from build123d import *

# Parameters (mm, degrees)
SKETCH_594_R           = 7.65
CUT_EXTRUDE_2199_DEPTH = 10
CHAMFER_START          = -4.9
CHAMFER_1_2_DEPTH      = 3.6500001
CHAMFER_START_2        = 1.2499999
CHAMFER_1_3_DEPTH      = 3.6500001
CHAMFER_START_3        = -5.4
CHAMFER_1_4_DEPTH      = 3
CHAMFER_START_4        = 2.4
CHAMFER_1_5_DEPTH      = 3
CHAMFER_START_5        = -2.4
CHAMFER_1_6_DEPTH      = 4.8


with BuildPart() as part:
    # Sketch 286 → Revolve 549 (revolve)
    with BuildSketch(Plane.XY, mode=Mode.PRIVATE) as revolve_549_sk:
        Polygon((0, 0), (7.65, 0), (7.65, 7), (9.15, 7), (9.15, 7.5), (7.65, 7.5), (7.65, 33.5), (0, 33.5), align=None)
    revolve(revolve_549_sk.sketch.rotate(Axis((0, 16.255686087, 0), (0, -1, 0)), 90), axis=Axis((0, 16.255686087, 0), (0, -1, 0)))

    # Sketch 594 → Cut-Extrude 2199 (cut)
    with BuildSketch(Plane(origin=(0, 33.5, 0), x_dir=(1, 0, 0), z_dir=(0, 1, 0))):
        with Locations(Location((0, 0, 0), (0, 0, 270))):
            Circle(SKETCH_594_R)
        with BuildLine():
            Line((-1.75, 2.4), (-1.75, 5.108571229))
            ThreePointArc((-1.75, 5.108571229), (0, 5.4), (1.75, 5.108571229))
            Line((1.75, 5.108571229), (1.75, 2.4))
            Line((1.75, 2.4), (4.837354649, 2.4))
            ThreePointArc((4.837354649, 2.4), (5.4, 0), (4.837354649, -2.4))
            Line((4.837354649, -2.4), (1.75, -2.4))
            Line((1.75, -2.4), (1.75, -5.108571229))
            ThreePointArc((1.75, -5.108571229), (0, -5.4), (-1.75, -5.108571229))
            Line((-1.75, -5.108571229), (-1.75, -2.4))
            Line((-1.75, -2.4), (-4.837354649, -2.4))
            ThreePointArc((-4.837354649, -2.4), (-5.4, 0), (-4.837354649, 2.4))
            Line((-4.837354649, 2.4), (-1.75, 2.4))
        make_face(mode=Mode.SUBTRACT)
    extrude(amount=-CUT_EXTRUDE_2199_DEPTH, mode=Mode.SUBTRACT)

    # Фаска1: read off the stored shape, not the designer's step
    # Фаска1 outline → Фаска1 (revolve, cut)
    with BuildSketch(Plane.XY):
        Polygon((5.4, 33.5), (4.9, 33.5), (5.4, 23.5), align=None)
    revolve(axis=Axis((0, 0, 0), (0, 1, 0)), mode=Mode.SUBTRACT)

    # Chamfer 1 2 outline → Chamfer 1 2 (cut)
    with BuildSketch(Plane.YZ.offset(CHAMFER_START)):
        Polygon((23.5, 2.4), (33.5, 1.9), (33.5, 2.4), align=None)
        Polygon((33.5, -2.4), (33.5, -1.9), (23.5, -2.4), align=None)
    extrude(amount=CHAMFER_1_2_DEPTH, mode=Mode.SUBTRACT)

    # Chamfer 1 3 outline → Chamfer 1 3 (cut)
    with BuildSketch(Plane.YZ.offset(CHAMFER_START_2)):
        Polygon((23.5, 2.4), (33.5, 1.9), (33.5, 2.4), align=None)
        Polygon((33.5, -2.4), (33.5, -1.9), (23.5, -2.4), align=None)
    extrude(amount=CHAMFER_1_3_DEPTH, mode=Mode.SUBTRACT)

    # Chamfer 1 4 outline → Chamfer 1 4 (cut)
    with BuildSketch(Plane.XY.offset(CHAMFER_START_3)):
        Polygon((1.75, 33.5), (1.249999967, 33.5), (1.75, 23.5), align=None)
        Polygon((-1.75, 23.5), (-1.25, 33.5), (-1.75, 33.5), align=None)
    extrude(amount=CHAMFER_1_4_DEPTH, mode=Mode.SUBTRACT)

    # Chamfer 1 5 outline → Chamfer 1 5 (cut)
    with BuildSketch(Plane.XY.offset(CHAMFER_START_4)):
        Polygon((1.75, 33.5), (1.249999967, 33.5), (1.75, 23.5), align=None)
        Polygon((-1.75, 23.5), (-1.25, 33.5), (-1.75, 33.5), align=None)
    extrude(amount=CHAMFER_1_5_DEPTH, mode=Mode.SUBTRACT)

    # Chamfer 1 6 outline → Chamfer 1 6 (add)
    with BuildSketch(Plane.XY.offset(CHAMFER_START_5)):
        Polygon((1.75, 23.5), (1.25, 33.5), (1.2499999, 23.5), align=None)
        Polygon((-1.2499999, 23.5), (-1.2499999, 33.5), (-1.75, 23.5), align=None)
    extrude(amount=CHAMFER_1_6_DEPTH)


solid = part.part
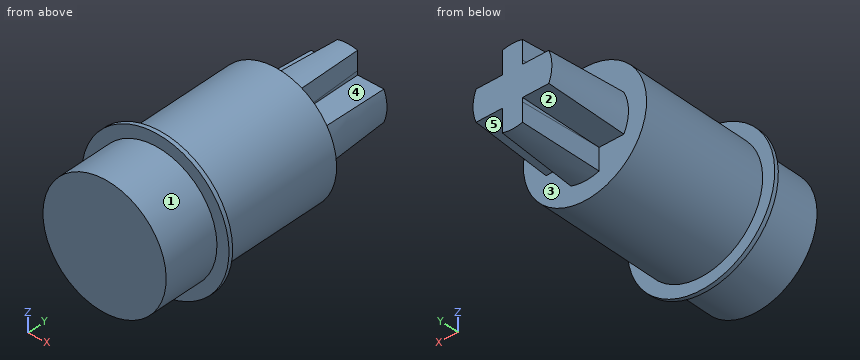
For this review, take the finished solid that the model builds, in its own axes (mm). Face numbers are marked on the shaded views. A direction names the side the tool comes from. Round coordinates to 2 decimals unless told otherwise and drop trailing zeros. Write each loop counter-clockwise with the first axis right and the second up, starting at its lowest first coordinate (ties: lowest second). Pieces come first, ordered by that corner, then holes. Notation, with made-up numbers: M 24,5 L 70,5 A23 cw 70,15 Z; hole C -25,-25.75 d6. An arc over 180 degrees is marked long. Write item = value, one per line. Start each with the question number.
(1) For the marked faces 1, 2, 3, 4 and 5, list the 3-axis set-ups (+Z, -Z, +X, -X, +Y, -Y) from which the entire face can be reached by the end or side of a thin tool; tool diameter is ignored.
(2) We need section D-D (x = -6.5). Give the boundary of the cut face in (y, z), then the cut area to 3 significant figures.
(3) We need section C-C (y = 14). Give the boundary of the cut face in (x, z).
(4) For line 1 along Y through (x, z) = (5.75, -2.25); line 2 along Y through (x, z) = (-4.75, 6.5); line 3 along Z through (x, y) = (-2.25, 27) (3 decimals), list the stretches that pass through material, from the lowest coordinate up.
(5) We need section A-A (z = 0). Give the boundary of the cut face in (x, y).
(6) Clearance check with flat-ended pins moving along their axes: pin 1 Ø1.5 at (x, y) = (-5, 6) entering from -Z; pin 2 Ø3 at (x, y) = (3, 16) entering from -Z; pin 3 Ø8 at (x, y) = (6, 26) entering from +Z; pin 4 Ø1.5 at (x, y) = (6, 28) entering from +Z. State where each tip first meets the part, or that it passes through.
(7) We need section B-B (x = 0). Give the boundary of the cut face in (y, z).
Results found:
q1.face_1 = -Y
q1.face_2 = -Z, -X, +Y
q1.face_3 = +Y
q1.face_4 = +Z, +X, +Y
q1.face_5 = -Z, +X, +Y
q2.outline = M 0,-4.03 L 7,-4.03 L 7,-6.44 L 7.5,-6.44 L 7.5,-4.03 L 23.5,-4.03 L 23.5,4.03 L 7.5,4.03 L 7.5,6.44 L 7,6.44 L 7,4.03 L 0,4.03 Z
q2.area = 192 mm²
q3.outline = C 0,0 d15.3
q4.line_1 = 0 to 23.5
q4.line_2 = 7 to 7.5
q4.line_3 = -2.225 to 2.225
q5.outline = M -9.15,7 L -7.65,7 L -7.65,0 L 7.65,0 L 7.65,7 L 9.15,7 L 9.15,7.5 L 7.65,7.5 L 7.65,23.5 L 5.4,23.5 L 4.9,33.5 L -4.9,33.5 L -5.4,23.5 L -7.65,23.5 L -7.65,7.5 L -9.15,7.5 Z
q6.pin_1 = -6.36
q6.pin_2 = -7.5
q6.pin_3 = 7.09
q6.pin_4 = through
q7.outline = M 0,-7.65 L 7,-7.65 L 7,-9.15 L 7.5,-9.15 L 7.5,-7.65 L 23.5,-7.65 L 23.5,-5.4 L 33.5,-4.9 L 33.5,4.9 L 23.5,5.4 L 23.5,7.65 L 7.5,7.65 L 7.5,9.15 L 7,9.15 L 7,7.65 L 0,7.65 Z
